Input: part model. Units: mm. Frame: model coordinates. Face numbers are marked on the shaded views. Give positions to 0.01 mm unless a question says otherwise; leave off trailing zeros. Loops run counter-clockwise (first coordinate to the right, second up) from the corner with the lowest first, then second, coordinate; pieces in that order, holes last. Notation, with made-up numbers: (-38, -36) -> (18, -36) arc R10 ccw to (18, -20) -> close; hole circle Ø2 at (68.5, -36.75). An arc over 180 degrees is marked (long way). One line per question, with ' | ' between items.
Autodesk Inventor part; units mm, degrees
ref_plane "YZ Plane" through (0, 0, 0) normal (1, 0, 0) x (0, 1, 0)
ref_plane "XZ Plane" through (0, 0, 0) normal (0, 1, 0) x (-1, 0, 0)
ref_plane "XY Plane" through (0, 0, 0) normal (0, 0, 1) x (1, 0, 0)
sketch "Sketch1" plane through (0, 0, 0) normal (0, 0, 1) x (1, 0, 0)
  line L0 (0, 0) -> (1.5, 0) construction
  line L1 (1.5, 0) -> (1.5, 1.5) construction
  line L2 (1.5, 1.5) -> (0, 1.5) construction
  line L3 (0, 0) -> (20, 0) construction
  line L4 (20, 0) -> (20, 1.5)
  line L5 (0, 0) -> (14.5, 0) construction
  line L6 (20, 1.5) -> (7.5, 1.5)
  line L7 (0, 1.5) -> (8.5, 1.5) construction
  line L8 (0, -1.5) -> (0, 9) construction
  line L9 (7.5, 1.5) -> (7.5, 7.5)
  line L10 (7.5, 7.5) -> (8.5, 7.5)
  line L11 (8.5, 7.5) -> (8.5, 2.5)
  line L12 (8.5, 2.5) -> (21, 2.5)
  line L13 (21, 2.5) -> (21, 0)
  line L14 (21, 0) -> (20, 0)
  line L15 (20, 0) -> (21, 0)
  line L16 (21, 0) -> (21, 0.5)
  line L17 (21, 0.5) -> (20, 0.5)
  line L18 (20, 0.5) -> (20, 0)
  dimension "d0" = 1.5
  dimension "d1" = 1.5
  dimension "d2" = 20
  dimension "d3" = 1.5
  dimension "d4" = 14.5
  dimension "d6" = 8.5
  dimension "d7" = 1
  dimension "d8" = 6
  dimension "d9" = 1
  dimension "d10" = 1
  dimension "d11" = 1
  dimension "d13" = 0.5
revolve "Revolution2" add sketch "Sketch1" angle 360 about axis through (0, -10, 0) along (0, 1, 0) contours L4 L6 L9 L10 L11 L12 L13 L17
properties part number "Seal_M"
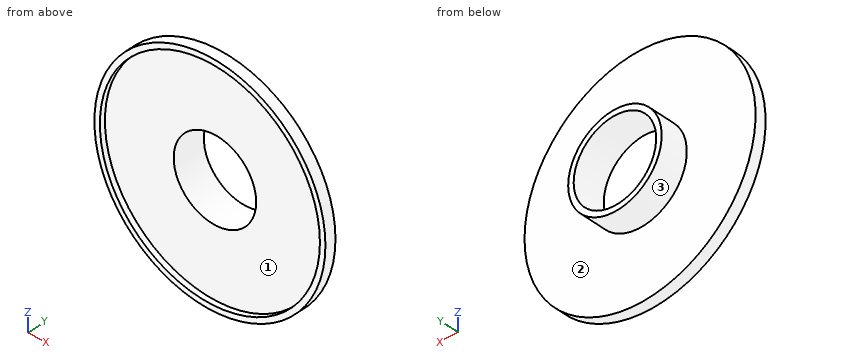
1. Section query A-A (x = 0). Output: boundary loops of the cut face in (y, z), then the cut area to 3 significant figures.
Determined:
outline: (0.5, -21) -> (2.5, -21) -> (2.5, -8.5) -> (7.5, -8.5) -> (7.5, -7.5) -> (1.5, -7.5) -> (1.5, -20) -> (0.5, -20) -> close; (0.5, 20) -> (1.5, 20) -> (1.5, 7.5) -> (7.5, 7.5) -> (7.5, 8.5) -> (2.5, 8.5) -> (2.5, 21) -> (0.5, 21) -> close | area: 39.0 mm2
2. Pull-direction query (Z, two-part tool) for the marked faces 1, 2 and 3; classes: pulls with the +Z half, pulls with the -Z half, needs draft (parallel to the pull), parting line crosses it, or undercut.
Determined:
face 1: undercut | face 2: needs draft | face 3: parting line crosses it
3. Ray query, line 1 along Z through (x, y) = (0, 3); line 2 along Z through (x, y) = (0, 0.8). Return the intervals inside material, ascending. Write a range as from..to.
Determined:
line 1: z = -8.5..-7.5, 7.5..8.5 | line 2: z = -21..-20, 20..21
4. Section query D-D (z = -9). Output: boundary loops of the cut face in (x, y), then the cut area to 3 significant figures.
Determined:
outline: (-18.97, 0.5) -> (-17.86, 0.5) -> (-17.86, 1.5) -> (17.86, 1.5) -> (17.86, 0.5) -> (18.97, 0.5) -> (18.97, 2.5) -> (-18.97, 2.5) -> close | area: 40.2 mm2
5. Pin query (flat end, axial travel): P1, Ø2, axis at x = 1.5, y = 6, coming from the +Z side; P2, Ø1, axis at y = 2, z = 1, coming from the -X side; P3, Ø5, axis at x = -7, z = -14, coming from the -Y side. Return the tip coordinate at first contact, or that it passes through.
Determined:
P1: stops at z = 8.49 | P2: stops at x = -20.99 | P3: stops at y = 1.5
6. Section query C-C (y = 3.75). Output: boundary loops of the cut face in (x, z), then the cut area to 3 significant figures.
Determined:
outline: circle Ø17 at (0, 0); hole circle Ø15 at (0, 0) | area: 50.3 mm2
7. Section query B-B (z = 0). Output: boundary loops of the cut face in (x, y), then the cut area to 3 significant figures.
Determined:
outline: (-21, 0.5) -> (-20, 0.5) -> (-20, 1.5) -> (-7.5, 1.5) -> (-7.5, 7.5) -> (-8.5, 7.5) -> (-8.5, 2.5) -> (-21, 2.5) -> close; (7.5, 1.5) -> (20, 1.5) -> (20, 0.5) -> (21, 0.5) -> (21, 2.5) -> (8.5, 2.5) -> (8.5, 7.5) -> (7.5, 7.5) -> close | area: 39.0 mm2
